The figure shows three views and two pictorial views of one solid part (mm, origin at its lowest corner). Answer the questions. Coordinates: 2 decimals unless noted, no trailing zeros. Write each loop counter-clockwise with the first axis right and the second up, starting at its lowest first coordinate (ties: lowest second). Pieces come first, ordered by that corner, then holes. Notation, with made-up numbers: M 62.25,28.5 L 67.25,28.5 A24 ccw 67.25,60.5 Z; hole C 36,22 d4. An arc over 180 degrees is marked long. Write item = value, one per line.
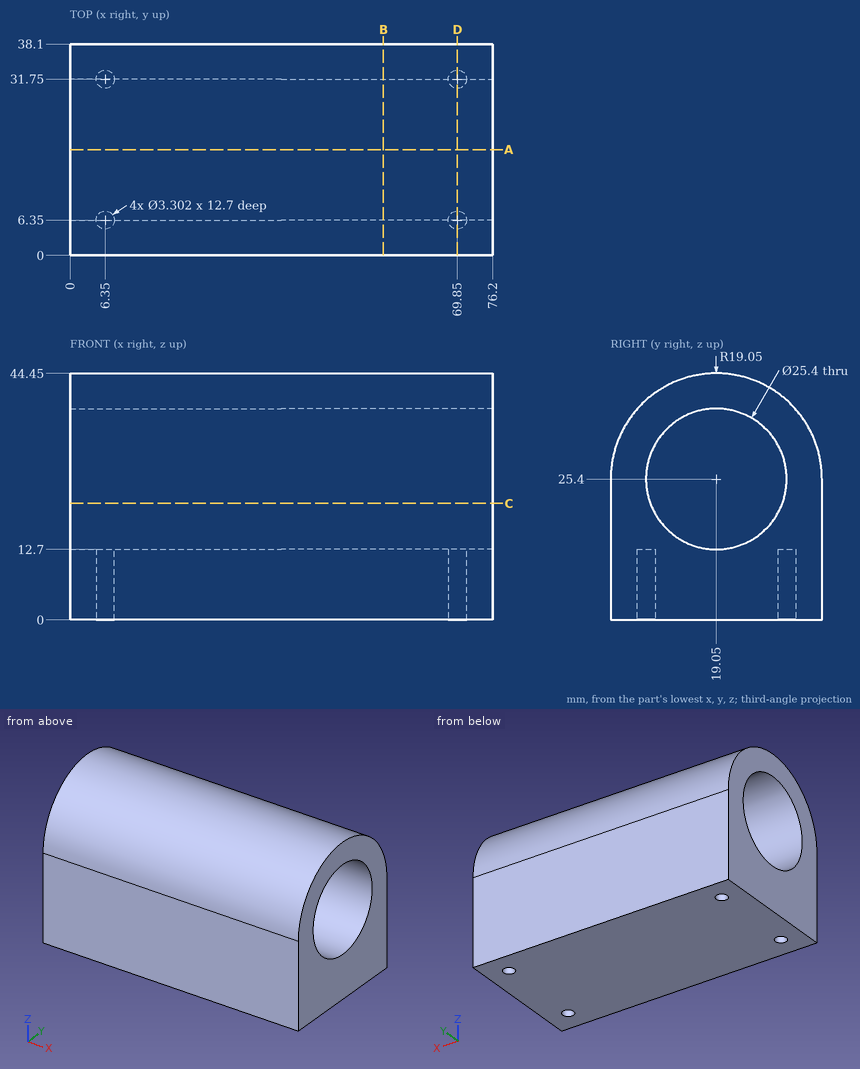
Item 1: Find section D-D (x = 69.85). Determine the outline of the cut face in (y, z).
Worked answers:
outline = M 0,0 L 4.7,0 L 4.7,12.7 L 8,12.7 L 8,0 L 30.1,0 L 30.1,12.7 L 33.4,12.7 L 33.4,0 L 38.1,0 L 38.1,25.4 A19.05 ccw 0,25.4 Z; hole C 19.05,25.4 d25.4
Item 2: Flat-ended cylindrical pins translate along their axes: pin 1 (4 mm diameter, centred on x = 6.35, y = 31.75, fed in from +Z); pin 2 (1 mm diameter, centred on x = 70.5, y = 32.5, fed in from -Z); pin 3 (10 mm diameter, centred on x = 13, y = 11, fed in from +Z); pin 4 (6 mm diameter, centred on y = 26, z = 26, fed in from +X). Find the tip coordinate at first contact, or state that the pin passes through.
Worked answers:
pin_1 = 41.16
pin_2 = 12.7
pin_3 = 44.2
pin_4 = through
Item 3: Consider line 1 along X through (y, z) = (31.75, 3.5); line 2 along Y through (x, z) = (69.85, 6.5); line 3 along X through (y, z) = (31, 3). Determine where each line is inside the solid, lowest interval first. Write a range as from..to.
Worked answers:
line_1 = 0..4.7, 8..68.2, 71.5..76.2
line_2 = 0..4.7, 8..30.1, 33.4..38.1
line_3 = 0..4.88, 7.82..68.38, 71.32..76.2
Item 4: Find section C-C (z = 21). Determine the outline of the cut face in (x, y), and give its area (3 significant figures).
Worked answers:
outline = M 0,0 L 76.2,0 L 76.2,7.14 L 0,7.14 Z; M 0,30.96 L 76.2,30.96 L 76.2,38.1 L 0,38.1 Z
area = 1,090 mm²
Item 5: Find section A-A (y = 19.05). Determine the outline of the cut face in (x, z), and give its area (3 significant figures).
Worked answers:
outline = M 0,0 L 76.2,0 L 76.2,12.7 L 0,12.7 Z; M 0,38.1 L 76.2,38.1 L 76.2,44.45 L 0,44.45 Z
area = 1,450 mm²
Item 6: Find section B-B (x = 56.5). Determine the outline of the cut face in (y, z), and give its area (3 significant figures).
Worked answers:
outline = M 0,0 L 38.1,0 L 38.1,25.4 A19.05 ccw 0,25.4 Z; hole C 19.05,25.4 d25.4
area = 1,030 mm²
